Autodesk Inventor part; units mm, degrees
ref_plane "YZ Plane" through (0, 0, 0) normal (1, 0, 0) x (0, 1, 0)
ref_plane "XZ Plane" through (0, 0, 0) normal (0, 1, 0) x (-1, 0, 0)
ref_plane "XY Plane" through (0, 0, 0) normal (0, 0, 1) x (1, 0, 0)
sketch "Sketch1" plane through (0, 0, 0) normal (0, 1, 0) x (-1, 0, 0)
  circle A0 centre (0, 0) radius 3
  circle A1 centre (0, 0) radius 60
  circle A2 centre (0, 0) radius 12.5
  circle A3 centre (0, 0) radius 45
  line L0 (0, -12.5) -> (0, -45)
  line L1 (0, 12.5) -> (0, 45)
  line L2 (-12.5, 0) -> (-45, 0)
  line L3 (12.5, 0) -> (45, 0)
  line L4 (0, 0) -> (5, 0) construction
  line L5 (-8.8388, -8.8388) -> (-31.8198, -31.8198)
  line L6 (8.8388, 8.8388) -> (31.8198, 31.8198)
  line L7 (0, 0) -> (40, 0) construction
  line L8 (-8.8388, 8.8388) -> (-31.8198, 31.8198)
  line L9 (8.8388, -8.8388) -> (31.8198, -31.8198)
  dimension "d4" = 25
  dimension "d5" = 90
  dimension "d0" = 6
  dimension "d1" = 120
  dimension "d7" = 45
extrude "Extrusion1" add sketch "Sketch1" along normal blind 10 contours A1 | A2 | L3 A3 L9 A2 | A2 L6 A3 L3 | A2 L1 A3 L6 | L9 A3 L0 A2 | A2 L8 A3 L1 | L0 A3 L5 A2 | A2 L2 A3 L8 | L5 A3 L2 A2
extrude "Extrusion2" cut sketch "Sketch1" along normal blind 10 contours L3 A3 L9 A2 | A2 L1 A3 L6 | L0 A3 L5 A2 | A2 L2 A3 L8
fillet "Fillet1" radius 3 2 edges at (60, 0, 0) (60, 10, 0)
fillet "Fillet2" radius 3 16 edges at (28.75, 0, 0) (20.3293, 0, 20.3293) (-20.3293, 0, 20.3293) (-28.75, 0, 0) (-20.3293, 0, -20.3293) (0, 0, -28.75) (20.3293, 0, -20.3293) (41.5746, 10, 17.2208) (20.3293, 10, -20.3293) (0, 10, -28.75) (-20.3293, 10, -20.3293) (-28.75, 10, 0) (-20.3293, 10, 20.3293) (0, 10, 28.75) (28.75, 10, 0) (0, 0, 28.75)
properties part number "roda_mdf"
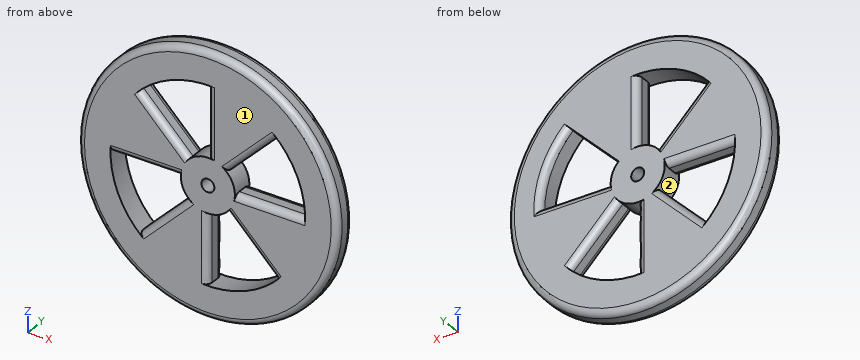
For this review, take the finished solid that the model builds, in its own axes (mm). Face numbers are marked on the shaded views. Coordinates: 2 decimals unless noted, no trailing zeros. Loops run counter-clockwise (first coordinate to the right, second up) from the corner with the lowest first, then second, coordinate; pieces in that order, holes last.
1. Insertion check: P1, Ø12, axis at x = -4, z = 18.5, coming from the +Y side; P2, Ø3, axis at x = -33.5, z = -38.5, coming from the -Y side; P3, Ø2, axis at x = -34, y = 4.5, coming from the -Z side; P4, Ø1.2, axis at x = 21, y = 5, coming from the +Z side. Each pin has a flat end and moves straight along its axis. Give the tip position at first contact, or say it passes through.
2. Mouldability with a two-part tool opening along X and no side actions: class the marked faces 1 and 2 as +X half, -X half, draft (parallel to the pull), parting line (faces both ways), or undercut.
3. For line 1 (Z direction, x = 0, y = 8.25); line 2 (X direction, y = 5, z = 31); line 3 (Z direction, x = 0, y = 8), list the stretches that pass through material, from the lowest coordinate up.
4. Add section A-A, the plane y = 5. Give the boundary of the cut face in (x, z), then the cut area to 3 significant figures.
5. Add section B-B, the plane x = 20. Count the separate pieces of the cut face and the enclosed holes in it, then the cut area to 3 significant figures.
Result:
1. P1: stops at y = 9.83
1. P2: stops at y = 0
1. P3: stops at z = -50.11
1. P4: stops at z = 56.43
2. face 1: draft
2. face 2: undercut
3. line 1: z = -59.73 to -45, -12.5 to -3, 3 to 12.5, 45 to 59.73
3. line 2: x = -51.37 to -31, 0 to 31, 32.62 to 51.37
3. line 3: z = -59.83 to -45, -12.5 to -3, 3 to 12.5, 45 to 59.83
4. outline: circle Ø120 at (0, 0); hole (-45, 0) arc R45 ccw to (-31.82, -31.82) - (-8.84, -8.84) arc R12.5 cw to (-12.5, 0) - close; hole (-31.82, 31.82) - (-8.84, 8.84) arc R12.5 cw to (0, 12.5) - (0, 45) arc R45 ccw to start; hole circle Ø6 at (0, 0); hole (0, -45) arc R45 ccw to (31.82, -31.82) - (8.84, -8.84) arc R12.5 cw to (0, -12.5) - close; hole (8.84, 8.84) arc R12.5 cw to (12.5, 0) - (45, 0) arc R45 ccw to (31.82, 31.82) - close
4. area: 8,350 mm2
5. separate pieces: 3
5. enclosed holes: 0
5. area: 708 mm2
